```python
from build123d import *

# Parameters (mm, degrees)
F0_W     = 71.067976
F0_H     = 32.185238
F0_R     = 7.020388
F1_DEPTH = 25.4


with BuildPart() as f1:
    # F0 (on Top) → F1 (new body)
    with BuildSketch(Plane.XY):
        Rectangle(F0_W, F0_H)
        with BuildLine():
            ThreePointArc((-35.533988, -16.092619), (0, -43.695065), (35.533988, -16.092619))
            Line((35.533988, -16.092619), (-35.533988, -16.092619))
        make_face()
        with Locations((0, -30.170137)):
            Circle(F0_R, mode=Mode.SUBTRACT)
    extrude(amount=F1_DEPTH)


solid = f1.part
```
Here's how the part is built. I have some questions about the finished solid (model axes, mm). Give positions to 0.01 mm unless a question says otherwise; leave off trailing zeros. Loops run counter-clockwise (first coordinate to the right, second up) from the corner with the lowest first, then second, coordinate; pieces in that order, holes last. Notation, with made-up numbers: M -36.5,-36.75 L 12.5,-36.75 A8 ccw 12.5,-26.75 Z; hole C -3.5,73.25 d10. An arc over 180 degrees is marked long. Put each result on its own line as item: value. Start each with the question number.
(1) I want a section at C-C on z = 11.5. Please give me the cut outline in (x, y).
(2) If we mould it in two halves opening along X, with no side actions, what happens to faces 1 (the flat face through (35.534, 0, 13)), 2 (the flat face through (0, -7, 0)), 3 (the cylindrical face through (-0.91, -23.21, 12.52))? For each: +X half, -X half, draft (parallel to the pull), parting line (faces both ways), or undercut.
(3) I need wall thicknesses on line 1 along Y through (x, z) = (0, 18.25); line 2 along Y through (x, z) = (5, 3.25); line 3 along X through (y, z) = (-30, 15). Which ranges of each line are inside material? Lowest first, please. Write a range as [from, to].
(4) I want a section at D-D on y = -18.5. Please give me the cut outline in (x, z).
(5) Will these pins go through, and if not, where does the flat tip stop? pin 1 Ø5 at (y, z) = (-24, 21) entering from -X; pin 2 Ø18.5 at (x, y) = (0, -30.17) entering from +Z; pin 3 Ø3 at (x, z) = (-20.5, 21.5) entering from -Y; pin 4 Ø12 at (y, z) = (-26.5, 19.5) entering from -X.
(6) I want a section at A-A on x = 0. Please give me the cut outline in (y, z).
(7) I want a section at B-B on y = -29. Please give me the cut outline in (x, z).
Answer block:
1. outline: M -35.53,-16.09 A36.67 ccw 35.53,-16.09 L 35.53,16.09 L -35.53,16.09 Z; hole C 0,-30.17 d14.04
2. face 1: +X half
2. face 2: draft
2. face 3: undercut
3. line 1: [-43.7, -37.19], [-23.15, 16.09]
3. line 2: [-43.35, -35.1], [-25.24, 16.09]
3. line 3: [-28.58, -7.02], [7.02, 28.58]
4. outline: M -34.83,0 L 34.83,0 L 34.83,25.4 L -34.83,25.4 Z
5. pin 1: x = -33.69
5. pin 2: z = 25.4
5. pin 3: y = -38.39
5. pin 4: x = -34.11
6. outline: M -43.7,0 L -37.19,0 L -37.19,25.4 L -43.7,25.4 Z; M -23.15,0 L 16.09,0 L 16.09,25.4 L -23.15,25.4 Z
7. outline: M -29.36,0 L -6.92,0 L -6.92,25.4 L -29.36,25.4 Z; M 6.92,0 L 29.36,0 L 29.36,25.4 L 6.92,25.4 Z
